CAD build for the part. Positions are in the model's coordinates, mm. A direction names the side the tool comes from. Round coordinates to 2 decimals unless told otherwise and drop trailing zeros. Loops run counter-clockwise (first coordinate to the right, second up) from the corner with the lowest first, then second, coordinate; pieces in that order, holes last. Notation, with made-up numbers: (-4.5, 20) -> (-0.5, 20) arc R7 ccw to (-0.5, 27) -> close; hole circle Ø11 at (65, 47). An arc over 180 degrees is marked (long way). Answer as CSV lines item,"result".
```python
from build123d import *

# Parameters (mm, degrees)
SKETCH1_R           = 85
BOSS_EXTRUDE2_DEPTH = 3
SKETCH2_R           = 82.5
BOSS_EXTRUDE3_DEPTH = 20
SKETCH3_R           = 50
CUT_EXTRUDE1_DEPTH  = 20
SKETCH9_R           = 4.7625
CUT_EXTRUDE9_DEPTH  = 19.05
SKETCH14_R          = 4.7625
CUT_EXTRUDE10_DEPTH = 19.05
CUT_EXTRUDE11_START = 19.05
SKETCH13_R          = 4.7625
CUT_EXTRUDE11_DEPTH = 19.05
CUT_EXTRUDE12_START = 19.05
SKETCH15_R          = 4.7625
CUT_EXTRUDE12_DEPTH = 19.05


with BuildPart() as part:
    # Sketch1 → Boss-Extrude2 (new body)
    with BuildSketch(Plane.XY):
        Circle(SKETCH1_R)
    extrude(amount=BOSS_EXTRUDE2_DEPTH)

    # Sketch2 → Boss-Extrude3 (add)
    with BuildSketch(Plane.XY.offset(3)):
        Circle(SKETCH2_R)
    extrude(amount=BOSS_EXTRUDE3_DEPTH)

    # Sketch3 → Cut-Extrude1 (cut)
    with BuildSketch(Plane.XY.offset(23)):
        Circle(SKETCH3_R)
    extrude(amount=-CUT_EXTRUDE1_DEPTH, mode=Mode.SUBTRACT)

    # Sketch9 → Cut-Extrude9 (cut)
    with BuildSketch(Plane(origin=(0, 82.5, 0), x_dir=(-1, 0, 0), z_dir=(0, -1, 0))):
        with Locations((0, -13)):
            Circle(SKETCH9_R)
    extrude(amount=CUT_EXTRUDE9_DEPTH, mode=Mode.SUBTRACT)

    # Sketch14 → Cut-Extrude10 (cut)
    with BuildSketch(Plane(origin=(82.5, 0, 0), x_dir=(0, 0, -1), z_dir=(1, 0, 0))):
        with Locations((-13, 0)):
            Circle(SKETCH14_R)
    extrude(amount=-CUT_EXTRUDE10_DEPTH, mode=Mode.SUBTRACT)

    # Sketch13 → Cut-Extrude11 (cut)
    with BuildSketch(Plane(origin=(0, -82.5, 0), x_dir=(1, 0, 0), z_dir=(0, 1, 0)).offset(CUT_EXTRUDE11_START)):
        with Locations(Location((0, -13, 0), (0, 0, 180))):
            Circle(SKETCH13_R)
    extrude(amount=-CUT_EXTRUDE11_DEPTH, mode=Mode.SUBTRACT)

    # Sketch15 → Cut-Extrude12 (cut)
    with BuildSketch(Plane(origin=(-82.5, 0, 0), x_dir=(0, 0, -1), z_dir=(1, 0, 0)).offset(CUT_EXTRUDE12_START)):
        with Locations((-13, 0)):
            Circle(SKETCH15_R)
    extrude(amount=-CUT_EXTRUDE12_DEPTH, mode=Mode.SUBTRACT)


solid = part.part
```
Q1. Drop flat-ended pins along their axis: pin 1 Ø10 at (x, y) = (-54.5, -8.5) entering from -Z; pin 2 Ø3 at (x, z) = (1.5, 12) entering from -Y; pin 3 Ø5 at (x, z) = (1.5, 13) entering from +Y; pin 4 Ø1 at (x, z) = (26, 8) entering from -Y. Give the stop position or say it passes through.
Results:
pin 1,"z = 0"
pin 2,"y = -63.45"
pin 3,"y = 63.45"
pin 4,"y = -78.46"
Q2. Slice it at D-D, the plane x = 24.5. Give the cut face in (y, z).
Results:
outline,"(-81.39, 0) -> (81.39, 0) -> (81.39, 3) -> (78.78, 3) -> (78.78, 23) -> (43.59, 23) -> (43.59, 3) -> (-43.59, 3) -> (-43.59, 23) -> (-78.78, 23) -> (-78.78, 3) -> (-81.39, 3) -> close"
Q3. Slice it at C-C, the plane z = 13. Give the cut face in (x, y), and give its area (3 significant figures).
Results:
outline,"(-82.36, -4.76) arc R82.5 ccw to (-4.76, -82.36) -> (-4.76, -63.45) -> (4.76, -63.45) -> (4.76, -82.36) arc R82.5 ccw to (82.36, -4.76) -> (63.45, -4.76) -> (63.45, 4.76) -> (82.36, 4.76) arc R82.5 ccw to (4.76, 82.36) -> (4.76, 63.45) -> (-4.76, 63.45) -> (-4.76, 82.36) arc R82.5 ccw to (-82.36, 4.76) -> (-63.45, 4.76) -> (-63.45, -4.76) -> close; hole circle Ø100 at (0, 0)"
area,"12,800 mm2"
Q4. Two-plate mould, pull along Y, no slides. Class faces 6 (the cylindrical face through (47.69, 15.02, 13.14)), 7 (the cylindrical face through (-67.453, -51.721, 1.479)), 8 (the flat face through (63.45, 0, 13)), 9 (the cylindrical face through (1.03, -72.84, 8.35)): pulls with the +Y half, pulls with the -Y half, needs draft (parallel to the pull), parting line crosses it, or undercut.
Results:
face 6,"undercut"
face 7,"parting line crosses it"
face 8,"undercut"
face 9,"needs draft"
Q5. Tool access for faces 1 (the cylindrical face through (-72.842, 1.431, 8.457)), 2 (the cylindrical face through (73.11, -4.65, 14.03)), 3 (the flat face through (0, -63.45, 13)), 4 (the cylindrical face through (0.62, 73.11, 8.28)), 5 (the flat face through (-1, 1, 3)): list every direction of +Z, -Z, +X, -X, +Y, -Y with a clear straight run to the whole face (end or side of a thin tool).
Results:
face 1,"-X"
face 2,"+X"
face 3,"-Y"
face 4,"+Y"
face 5,"+Z"
Q6. Probe L1, parallel to Z at x = 0, y = 74; L2, parallel to X at y = 9, z = 6.25; L3, parallel to X at y = 13, z = 12.5. List the from-to ranges inside material, lowest first. Write a range as [from, to].
Results:
L1,"[0, 8.24], [17.76, 23]"
L2,"[-82.01, -49.18], [49.18, 82.01]"
L3,"[-81.47, -48.28], [48.28, 81.47]"
Q7. Slice it at A-A, the plane y = 0. Give the cut face in (x, z).
Results:
outline,"(-85, 0) -> (85, 0) -> (85, 3) -> (82.5, 3) -> (82.5, 8.24) -> (63.45, 8.24) -> (63.45, 17.76) -> (82.5, 17.76) -> (82.5, 23) -> (50, 23) -> (50, 3) -> (-50, 3) -> (-50, 23) -> (-82.5, 23) -> (-82.5, 17.76) -> (-63.45, 17.76) -> (-63.45, 8.24) -> (-82.5, 8.24) -> (-82.5, 3) -> (-85, 3) -> close"
